Read the model definition and answer for the solid it produces. Units are mm, in the model's axes. A direction names the side the tool comes from. Coordinates: 2 decimals unless noted, no trailing zeros. Order: outer loops, then holes, each group sorted by start corner. A loop starts at its lowest first (then second) coordinate and runs counter-clockwise, first axis right, second up. Notation, with made-up numbers: M -22.75,58.5 L 32.25,58.5 A35 ccw 32.25,97.5 Z; hole C 4.5,8 d10. An arc over 180 degrees is marked long. One line per question, with ' | ' between items. Start each with the question number.
1) A tool of negligible diameter and unlimited length cuts with its end or side. For faces 1 (the face through (-33, 0, 25)), 2 (the face through (-1, 40, 7)), 3 (the face through (30.58, 22.063, 7.22)), from which of +Z, -Z, +X, -X, +Y, -Y can it reach the whole face along a straight path? Write none if from no direction.
2) Find section A-A, the plane y = 19. Write down the section's boundary in (x, z).
3) Find section D-D, the plane z = 16.5. Write down the section's boundary in (x, y).
4) Find section C-C, the plane y = 5. Write down the section's boundary in (x, z).
5) Find section B-B, the plane x = 0. Write down the section's boundary in (y, z).
6) Consider probe 1 along X at (y, z) = (0, 38); probe 2 along Z at (x, y) = (3.5, 24.5); probe 3 along X at (y, z) = (2, 4). Determine where each line is inside the solid, lowest interval first.
7) The mould has two halves that part along Y. Classify faces 4 (the face through (-1, 20, 14.645)), 5 (the face through (-3.252, -14.643, 24.65)), 6 (the face through (32, 0, 25)): +Y half, -Y half, draft (parallel to the pull), parting line (faces both ways), or undercut.
8) Given P1, Ø10, axis at x = 39.5, z = 22.5, coming from the +Y side, flat-ended and moving along its own axis, determine where the tip first touches the part or whether it passes through.
from build123d import *

# Parameters (mm, degrees)
F0_W     = 100
F0_H     = 80
F0_R     = 15
F1_DEPTH = 50
F2_W     = 132.103257
F2_H     = 19.725826
F3_DEPTH = 50
F4_R     = 5
F5_DEPTH = 25


with BuildPart() as f1:
    # F0 (on Top) → F1 (new body)
    with BuildSketch(Plane.XY):
        Rectangle(F0_W, F0_H)
        Circle(F0_R, mode=Mode.SUBTRACT)
    extrude(amount=F1_DEPTH)

    # F2 (on Front) → F3 (cut)
    with BuildSketch(Plane.XZ):
        with Locations((2.241571, 24.507845)):
            Rectangle(F2_W, F2_H)
    extrude(amount=-F3_DEPTH, mode=Mode.SUBTRACT)

    # F4 (on Top) → F5 (cut)
    with BuildSketch(Plane.XY):
        with Locations((31.663418, 26.944561)):
            Circle(F4_R)
    extrude(amount=F5_DEPTH, mode=Mode.SUBTRACT)


solid = f1.part
Report:
1) face 1: +X, -X, +Y | face 2: +Z, -Z, +X, -X, +Y | face 3: -Z
2) outline: M -50,0 L 50,0 L 50,14.64 L -50,14.64 Z; M -50,34.37 L 50,34.37 L 50,50 L -50,50 Z
3) outline: M -50,-40 L 50,-40 L 50,0 L 15,0 A15 cw -15,0 L -50,0 Z
4) outline: M -50,0 L -14.14,0 L -14.14,14.64 L -50,14.64 Z; M -50,34.37 L -14.14,34.37 L -14.14,50 L -50,50 Z; M 14.14,0 L 50,0 L 50,14.64 L 14.14,14.64 Z; M 14.14,34.37 L 50,34.37 L 50,50 L 14.14,50 Z
5) outline: M -40,0 L -15,0 L -15,50 L -40,50 Z; M 15,0 L 40,0 L 40,14.64 L 15,14.64 Z; M 15,34.37 L 40,34.37 L 40,50 L 15,50 Z
6) probe 1: x = -50 to -15, 15 to 50 | probe 2: z = 0 to 14.64, 34.37 to 50 | probe 3: x = -50 to -14.87, 14.87 to 50
7) face 4: draft | face 5: undercut | face 6: +Y half
8) P1: stops at y = 0
